```python
from build123d import *

# Parameters (mm, degrees)
F0_W     = 20
F0_H     = 5
F0_R     = 2
F1_DEPTH = 1.5
F2_W     = 3.5
F2_H     = 2
F3_DEPTH = 8
F4_W     = 13
F4_H     = 2
F5_DEPTH = 3


with BuildPart() as f1:
    # F0 (on Top) → F1 (new body)
    with BuildSketch(Plane.XY):
        Rectangle(F0_W, F0_H)
        with BuildLine():
            ThreePointArc((-10, -2.5), (0, -12.5), (10, -2.5))
            Line((10, -2.5), (-10, -2.5))
        make_face()
        with Locations((0, -7.5)):
            Circle(F0_R, mode=Mode.SUBTRACT)
    extrude(amount=F1_DEPTH)

    # F2 (on face) → F3 (join)
    with BuildSketch(Plane.XY.offset(1.5)):
        with Locations((-8.25, 1.5)):
            Rectangle(F2_W, F2_H)
        with Locations((8.25, 1.5)):
            Rectangle(F2_W, F2_H)
    extrude(amount=F3_DEPTH)

    # F4 (on face) → F5 (join)
    with BuildSketch(Plane.XY.offset(1.5)):
        with Locations((0, 1.5)):
            Rectangle(F4_W, F4_H)
    extrude(amount=F5_DEPTH)


solid = f1.part
```
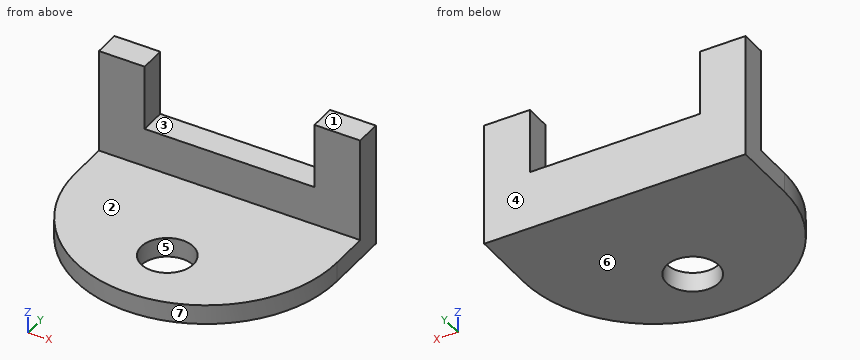
Verification items for the finished model (mm, model axes). Face numbers are marked on the shaded views. A direction names the side the tool comes from. Coordinates: 2 decimals unless noted, no trailing zeros. Loops run counter-clockwise (first coordinate to the right, second up) from the corner with the lowest first, then second, coordinate; pieces in that order, holes last. Notation, with made-up numbers: (42, 46.5) -> (79, 46.5) arc R6 cw to (79, 56.5) -> close; hole circle Ø6 at (22, 34.5). An arc over 180 degrees is marked (long way). Answer in a Markdown table with one row per item.
1) Depth check by flat-ended pin: P1, Ø2, axis at x = 3, y = 1.5, coming from the +Z side; P2, Ø3, axis at x = 2, y = -9.5, coming from the +Z side. Enter the tip coordinate at first touch or a pass-through.
The answers:
| item | result |
|---|---|
| P1 | stops at z = 4.5 |
| P2 | stops at z = 1.5 |
2) Draft check along Y on the marked faces 4, 5, 6 and 7. Enter one of: released by +Y, released by -Y, zero draft, split by the parting line, or undercut.
The answers:
| item | result |
|---|---|
| face 4 | released by +Y |
| face 5 | undercut |
| face 6 | zero draft |
| face 7 | released by -Y |
3) Access from +Z, -Z, +X, -X, +Y, -Y to the whole of each face (thin tool, end or side, straight path). Record for the marked faces 1, 2 and 3.
The answers:
| item | result |
|---|---|
| face 1 | +Z, +X, -X, +Y, -Y |
| face 2 | +Z, +X, -X, -Y |
| face 3 | +Z, +Y, -Y |
4) Section check A-A (z = 8.25). Record the cut outline in (x, y).
The answers:
| item | result |
|---|---|
| outline | (-10, 0.5) -> (-6.5, 0.5) -> (-6.5, 2.5) -> (-10, 2.5) -> close; (6.5, 0.5) -> (10, 0.5) -> (10, 2.5) -> (6.5, 2.5) -> close |
5) Scan lines: line 1 along Y through (x, z) = (0, 0.4); line 2 along Z through (x, y) = (-2.5, -6.5); line 3 along Y through (x, z) = (-6.75, 4.75). Record each from-to range of solid material in increasing order. Write a range as from..to.
The answers:
| item | result |
|---|---|
| line 1 | y = -12.5..-9.5, -5.5..2.5 |
| line 2 | z = 0..1.5 |
| line 3 | y = 0.5..2.5 |
6) Section check D-D (y = 0.75). Record the cut outline in (x, z).
The answers:
| item | result |
|---|---|
| outline | (-10, 0) -> (10, 0) -> (10, 9.5) -> (6.5, 9.5) -> (6.5, 4.5) -> (-6.5, 4.5) -> (-6.5, 9.5) -> (-10, 9.5) -> close |
7) Section check B-B (x = 0). Record the cut outline in (y, z), and give its area (3 significant figures).
The answers:
| item | result |
|---|---|
| outline | (-12.5, 0) -> (-9.5, 0) -> (-9.5, 1.5) -> (-12.5, 1.5) -> close; (-5.5, 0) -> (2.5, 0) -> (2.5, 4.5) -> (0.5, 4.5) -> (0.5, 1.5) -> (-5.5, 1.5) -> close |
| area | 22.5 mm2 |
8) Section check C-C (y = -5.75). Record the cut outline in (x, z).
The answers:
| item | result |
|---|---|
| outline | (-9.46, 0) -> (-0.97, 0) -> (-0.97, 1.5) -> (-9.46, 1.5) -> close; (0.97, 0) -> (9.46, 0) -> (9.46, 1.5) -> (0.97, 1.5) -> close |
